Input: part model. Units: mm. Frame: model coordinates. A direction names the side the tool comes from. Coordinates: 2 decimals unless noted, no trailing zeros. Write each loop counter-clockwise with the first axis right and the second up, starting at its lowest first coordinate (ties: lowest second). Pieces come first, ordered by that corner, then holes. Notation, with made-up numbers: M 61,23.5 L 98,23.5 A34 ccw 98,61.5 Z; hole C 19,-36 d7. An arc over 180 degrees is marked long. Use one line per item in the form item = value.
from build123d import *

# Parameters (mm, degrees)
SKETCH1_R                = 1.75
BOSS_EXTRUDE1_DEPTH      = 1.5
BOSS_EXTRUDE2_DEPTH      = 84
BOSS_EXTRUDE3_DEPTH      = 1.5
BOSS_EXTRUDE3_DEPTH_BACK = 1.5
BOSS_EXTRUDE4_DEPTH      = 2
SKETCH5_R                = 1.75
CUT_EXTRUDE1_DEPTH       = 2
CUT_EXTRUDE2_DEPTH       = 150.007183132
CUT_EXTRUDE2_DEPTH_BACK  = 150.007183132
SKETCH6_W                = 84
SKETCH6_H                = 11.5
BOSS_EXTRUDE6_START      = -2
SKETCH7_W                = 3
SKETCH7_H                = 4
BOSS_EXTRUDE6_DEPTH      = 2.5
FILLET1_R                = 2
CHAMFER1_SIZE            = 1
FILLET2_R                = 8
SKETCH8_W                = 26
SKETCH8_H                = 23
CUT_EXTRUDE3_DEPTH       = 22.4262221


with BuildPart() as part:
    # Sketch1 → Boss-Extrude1 (new body)
    with BuildSketch(Plane.XY):
        with BuildLine():
            Line((-38.75, -134.5), (38.75, -134.5))
            Line((38.75, -134.5), (42, -134.5))
            Line((42, -134.5), (42, -132.48653227))
            ThreePointArc((42, -132.48653227), (43.775, -129.5), (42, -126.51346773))
            Line((42, -126.51346773), (42, -6.48653227))
            ThreePointArc((42, -6.48653227), (43.741212037, -3.021861398), (41.104087703, -0.179091823))
            Line((41.104087703, -0.179091823), (42, 0))
            Line((42, 0), (-41, 0))
            Line((-41, 0), (-41.193033114, -0.199875483))
            ThreePointArc((-41.193033114, -0.199875483), (-43.747330957, -3.067121364), (-42, -6.48653227))
            Line((-42, -6.48653227), (-42, -126.51346773))
            ThreePointArc((-42, -126.51346773), (-43.775, -129.5), (-42, -132.48653227))
            Line((-42, -132.48653227), (-42, -134.5))
            Line((-42, -134.5), (-38.75, -134.5))
        make_face()
        with Locations((-40.375, -129.5)):
            Circle(SKETCH1_R, mode=Mode.SUBTRACT)
        with Locations((40.375, -129.5)):
            Circle(SKETCH1_R, mode=Mode.SUBTRACT)
        with Locations((40.375, -3.5)):
            Circle(SKETCH1_R, mode=Mode.SUBTRACT)
        with Locations((-40.375, -3.5)):
            Circle(SKETCH1_R, mode=Mode.SUBTRACT)
    extrude(amount=BOSS_EXTRUDE1_DEPTH)

    # Sketch2 → Boss-Extrude2 (add)
    with BuildSketch(Plane.ZY.offset(42)):
        Polygon((1.5, -134.5), (1.5, -136.7), (-40, -136.7), (-40, -134.7), (0, -134.7), (0, -134.5), (0, -132.48653227), (1.5, -132.48653227), align=None)
    extrude(amount=-BOSS_EXTRUDE2_DEPTH)

    # Sketch3 → Boss-Extrude3 (add, two sides: drawn at the far end of the back side and taken through both)
    with BuildSketch(Plane(origin=(-15, 0, 0), x_dir=(0, 0, -1), z_dir=(1, 0, 0)).offset(-BOSS_EXTRUDE3_DEPTH_BACK)):
        Polygon((0, -119.7), (15, -134.7), (0, -134.7), align=None)
    extrude(amount=BOSS_EXTRUDE3_DEPTH + BOSS_EXTRUDE3_DEPTH_BACK)

    # Sketch4 → Boss-Extrude4 (add)
    with BuildSketch(Plane.XZ.offset(136.7)):
        with BuildLine():
            Line((-42, -17.01346773), (-42, -22.98653227))
            ThreePointArc((-42, -22.98653227), (-43.775, -20), (-42, -17.01346773))
        make_face()
        with BuildLine():
            Line((42, -17.01346773), (42, -22.98653227))
            ThreePointArc((42, -22.98653227), (43.775, -20), (42, -17.01346773))
        make_face()
    extrude(amount=-BOSS_EXTRUDE4_DEPTH)

    # Sketch5 → Cut-Extrude1 (cut)
    with BuildSketch(Plane.XZ.offset(136.7)):
        with Locations(Location((40.375, -20, 0), (0, 0, 270))):
            Circle(SKETCH5_R)
        with Locations(Location((-40.375, -20, 0), (0, 0, 270))):
            Circle(SKETCH5_R)
    extrude(amount=-CUT_EXTRUDE1_DEPTH, mode=Mode.SUBTRACT)

    # Sketch6 → Cut-Extrude2 (cut, two sides: drawn at the far end of the back side and taken through both)
    with BuildSketch(Plane.XZ.offset(136.7).offset(-CUT_EXTRUDE2_DEPTH_BACK)):
        with Locations((0, -34.25)):
            Rectangle(SKETCH6_W, SKETCH6_H)
    extrude(amount=CUT_EXTRUDE2_DEPTH + CUT_EXTRUDE2_DEPTH_BACK, mode=Mode.SUBTRACT)

    # Sketch7 → Boss-Extrude6 (add)
    with BuildSketch(Plane.XZ.offset(136.7).offset(BOSS_EXTRUDE6_START)):
        with Locations((-37.3, -26.5)):
            Rectangle(SKETCH7_W, SKETCH7_H)
        with Locations((37.3, -26.5)):
            Rectangle(SKETCH7_W, SKETCH7_H)
    extrude(amount=-BOSS_EXTRUDE6_DEPTH)

    # Fillet1
    fillet1_edges = [part.edges().sort_by_distance(p)[0] for p in [
        (42, -135.7, -28.5),
        (-42, -135.7, -28.5),
    ]]
    fillet(fillet1_edges, radius=FILLET1_R)

    # Chamfer1
    chamfer1_edges = [part.edges().sort_by_distance(p)[0] for p in [
        (-37.3, -134.7, -24.5),
        (-37.3, -132.2, -24.5),
        (37.3, -134.7, -24.5),
        (37.3, -132.2, -24.5),
    ]]
    chamfer(chamfer1_edges, length=CHAMFER1_SIZE)

    # Fillet2
    # the kernel refuses this fillet: 8 mm, written as the material it takes off along each edge
    with BuildSketch(Plane(origin=(-30.803909917, -133.2, -24.5), x_dir=(0, -1.0, -1.118394266079786e-11), z_dir=(-1, 0, 0))) as fillet2_piece_1:
        with BuildLine():
            CenterArc((4.243746579, -7.06996192), FILLET2_R, 117.902496562, 17.097503438)
            Line((-1.413107671, -1.413107671), (0, 0))
            Line((0, 0), (0.5, 0))
        make_face()
    extrude(amount=12.992180166, mode=Mode.SUBTRACT)
    with BuildSketch(Plane(origin=(30.803909917, -133.2, -24.5), x_dir=(0, 0.7071067811865501, -0.7071067811865448), z_dir=(1, 0, 0))) as fillet2_piece_2:
        with BuildLine():
            CenterArc((1.998436033, -8), FILLET2_R, 90, 17.097503438)
            Line((-0.353553391, -0.353553391), (0, 0))
            Line((0, 0), (1.998436033, 0))
        make_face()
    extrude(amount=12.992180166, mode=Mode.SUBTRACT)

    # Sketch8 → Cut-Extrude3 (cut)
    with BuildSketch(Plane.XZ.offset(136.7)):
        with Locations((3, -14)):
            Rectangle(SKETCH8_W, SKETCH8_H)
    extrude(amount=-CUT_EXTRUDE3_DEPTH, mode=Mode.SUBTRACT)


solid = part.part
(1) Pull-direction query (Z, two-part tool) for faces 1 (the flat face through (-1, -135, -28.5)), 2 (the flat face through (-1, -69, 1.5)), 3 (the cylindrical face through (38.667, -135.714, -19.621)), 4 (the flat face through (-13.5, -130, -4)); classes: pulls with the +Z half, pulls with the -Z half, needs draft (parallel to the pull), parting line crosses it, or undercut.
Computed:
face_1 = pulls with the -Z half
face_2 = pulls with the +Z half
face_3 = undercut
face_4 = needs draft
(2) Section query C-C on x = -8.5. Return the cut outline in (y, z).
Computed:
outline = M -136.7,-28.5 L -134.7,-28.5 L -134.7,-25.5 L -136.7,-25.5 Z; M -136.7,-2.5 L -134.7,-2.5 L -134.7,0 L 0,0 L 0,1.5 L -136.7,1.5 Z
(3) First-contact query: pin 1 Ø4.5 at (x, y) = (40.375, -3.5) entering from -Z; pin 2 Ø2 at (x, z) = (-40.375, -20) entering from +Y; pin 3 Ø1.3 at (y, z) = (-133, -26.5) entering from +X; pin 4 Ø1 at (y, z) = (-135, -25.5) entering from +X. Flat tips, straight axial feed; report the tip coordinate or a pass-through.
Computed:
pin_1 = 0
pin_2 = through
pin_3 = 38.8
pin_4 = 42
(4) Section query B-B on y = -129.5. Return the cut outline in (x, z) (3 decimals), plus the area to 3 significant figures.
Computed:
outline = M -43.775,0 L -42.125,0 L -42.125,1.5 L -43.775,1.5 Z; M -38.625,0 L -16.5,0 L -16.5,-9.8 L -13.5,-9.8 L -13.5,0 L 38.625,0 L 38.625,1.5 L -38.625,1.5 Z; M 42.125,0 L 43.775,0 L 43.775,1.5 L 42.125,1.5 Z
area = 150 mm^2
(5) Line query: probe 1 along X at (y, z) = (-129.5, 0.8) (3 decimals); probe 2 along Z at (x, y) = (1, -63); probe 3 along Y at (x, z) = (37.5, -19). Output: solid intervals per line, ascending.
Computed:
probe_1 = -43.775 to -42.125, -38.625 to 38.625, 42.125 to 43.775
probe_2 = 0 to 1.5
probe_3 = -136.7 to -134.7
(6) Section query A-A on z = -20. Return the cut outline in (x, y) (3 decimals), plus the area to 3 significant figures.
Computed:
outline = M -43.775,-136.7 L -42.125,-136.7 L -42.125,-134.7 L -43.775,-134.7 Z; M -38.625,-136.7 L -10,-136.7 L -10,-134.7 L -38.625,-134.7 Z; M 16,-136.7 L 38.625,-136.7 L 38.625,-134.7 L 16,-134.7 Z; M 42.125,-136.7 L 43.775,-136.7 L 43.775,-134.7 L 42.125,-134.7 Z
area = 109 mm^2
(7) Section query D-D on z = -12. Return the cut outline in (x, y), plus the area to 3 significant figures.
Computed:
outline = M -42,-136.7 L -10,-136.7 L -10,-134.7 L -13.5,-134.7 L -13.5,-131.7 L -16.5,-131.7 L -16.5,-134.7 L -42,-134.7 Z; M 16,-136.7 L 42,-136.7 L 42,-134.7 L 16,-134.7 Z
area = 125 mm^2
(8) Set-up query: faces 5 (the flat face through (-16.5, -130, -4)), 6 (the flat face through (-42, -136, -8)), 7 (the flat face through (37, -132.2, -27)), 8 (the flat face through (42, -136, -8)), 9 (the flat face through (-35.8, -133, -27)). Return all of +Z, -Z, +X, -X, +Y, -Y with unobstructed straight access to the full face (end or side cutting, diameter ignored); none if empty.
Computed:
face_5 = -Z, -X, +Y
face_6 = +Z, -X, -Y
face_7 = -Z, +X, -X, +Y
face_8 = +Z, +X, -Y
face_9 = -Z, +Y
